Autodesk Inventor part; units mm, degrees
ref_plane "MSC_PF1" through (0, 0, 0) normal (1, 0, 0) x (0, 1, 0)
ref_plane "MSC_PT1" through (0, 0, 0) normal (0, 0, -1) x (-1, 0, 0)
ref_plane "YZ Plane" through (0, 0, 0) normal (1, 0, 0) x (0, 1, 0)
sketch "Sketch1" plane through (0, 0, 0) normal (0, 1, 0) x (-1, 0, 0)
  point P0 (0, 0)
sketch "Sketch2" plane through (0, 0, 0) normal (0, 1, 0) x (-1, 0, 0)
  line L0 (-3, -20) -> (0, -20)
  line L1 (-3, -3.3) -> (-3, -20)
  line L2 (-6, -0.3) -> (-3, -3.3)
  line L3 (-6, 0) -> (-6, -0.3)
  line L4 (0, 0) -> (-6, 0)
  line L5 (0, -20) -> (0, 0)
  line L6 (0, -20) -> (0, 0)
  line L7 (0, -24) -> (0, 4)
  line L8 (1.2, 0) -> (-7.2, 0)
  dimension "d3" = 6
  dimension "d5" = 3
  dimension "d7" = 20
  dimension "ParC" = 0.3
  dimension "d22" = 0
  dimension "d23" = 0
  dimension "d43" = 45
revolve "Revolution1" add sketch "Sketch2" angle 360 about axis through (0, 0, -20) along (0, 0, -1)
sketch "Sketch3" plane through (0, 0, 0) normal (0, 0, 1) x (1, 0, 0)
  line L0 (-2, 1.1547) -> (-2, -1.1547)
  line L1 (0, 2.3094) -> (-2, 1.1547)
  line L2 (2, 1.1547) -> (0, 2.3094)
  line L3 (2, -1.1547) -> (2, 1.1547)
  line L4 (0, -2.3094) -> (2, -1.1547)
  line L5 (-2, -1.1547) -> (0, -2.3094)
  circle A0 centre (0, 0) radius 2 construction
  circle A1 centre (0, 0) radius 3 construction
  dimension "d11" = 4
  dimension "d13" = 120
  dimension "d15" = 120
extrude "Extrusion1" cut sketch "Sketch3" against normal blind 2.5
fillet "Fillet1" radius 0.3 1 edges at (-3, 0, -3.3)
chamfer "Chamfer1" distance 0.5 angle 45 1 edges at (-3, 0, -20) measured on face at (2.4612, -1.7154, -14.4748)
thread "Thread1"
ref_plane "MSC_PF1" through (0, 0, 0) normal (1, 0, 0) x (0, 1, 0)
ref_plane "MSC_PT1" through (0, 0, 0) normal (0, 0, -1) x (-1, 0, 0)
equation "\"d3\" = 0.5 * dk"
equation "\"d5\" = 0.5 * NND"
equation "\"d43\" = 0.5 * ang"
equation "\"d18\" = r"
equation "\"d19\" = 0.5 * PTC"
equation "\"d39\" = 0.5 * PTC"
equation "\"d11\" = ParS"
equation "\"d16\" = ParT"
equation "\"NND\" = 6"
equation "\"PTC\" = 1"
equation "\"dk\" = 12"
equation "\"ParK\" = 3.3"
equation "\"ParS\" = 4"
equation "\"ParT\" = 2.5"
equation "\"r\" = 0.3"
equation "\"NLG\" = 25"
equation "\"ang\" = 90deg"
equation "\"THREADDIA\" = NND"
properties part number "CSK Allen Key 6x20mm" material "Steel, Mild"
Geometry: final body of the model. Coordinates: model frame, mm. A direction names the side the tool comes from. Round coordinates to 2 decimals unless told otherwise and drop trailing zeros. Loops run counter-clockwise (first coordinate to the right, second up) from the corner with the lowest first, then second, coordinate; pieces in that order, holes last.
Q1. Section A-A on z = -1.5. Return loops of the section in (x, y), plus the area to 3 significant figures.
Q2. Access query for faces 5 (the cylindrical face through (-3, 0, -12)), 6 (the flat face through (-0.99, 1.74, -1.23)), 7 (the flat face through (3, 0, 0)). Directions: +Z, -Z, +X, -X, +Y, -Y. A direction counts if a zero-diameter tool reaches every point of the face in a straight line with its end or side. Return the directions, or none.
Q3. Pin query (flat end, axial travel): P1, Ø4, axis at y = -1.5, z = -11, coming from the +X side; P2, Ø5, axis at y = 0.5, z = -9.5, coming from the -X side; P3, Ø4, axis at x = 0.5, z = -6, coming from the -Y side. Return the tip coordinate at first contact, or that it passes through.
Q4. Material intervals for L1, parallel to Z at x = 0.75, y = 1; L2, parallel to Y at x = 0, z = -9.25; L3, parallel to X at y = -2.5, z = -16.25, sorted ascending.
Q5. Pull-direction query (Y, two-part tool) for faces 1 (the flat face through (-1.014, -1.724, -1.232)), 2 (the flat face through (0, 0, -20)), 3 (the flat face through (-2, 0, -1)), 4 (the cylindrical face through (-4.42, -4.06, -0.15)); classes: released by +Y, released by -Y, zero draft, split by the parting line, or undercut.
Q6. Section B-B on z = -5. Return loops of the section in (x, y).
Evaluation:
1. outline: circle Ø9.6 at (0, 0); hole (-2, -1.15) - (0, -2.31) - (2, -1.15) - (2, 1.15) - (0, 2.31) - (-2, 1.15) - close
1. area: 58.5 mm2
2. face 5: -Z
2. face 6: +Z
2. face 7: +Z, +X, -X, +Y, -Y
3. P1: stops at x = 3
3. P2: stops at x = -3
3. P3: stops at y = -3
4. L1: z = -20 to -2.5
4. L2: y = -3 to 3
4. L3: x = -1.66 to 1.66
5. face 1: undercut
5. face 2: zero draft
5. face 3: undercut
5. face 4: split by the parting line
6. outline: circle Ø6 at (0, 0)
